Can you work these out from the drawing? Everything is in mm from the part's minimum corner. A direction names the side the tool comes from. Round coordinates to 2 decimals unless told otherwise and drop trailing zeros. Order: outer loops, then holes, each group sorted by start corner. A loop starts at its lowest first (then second) coordinate and runs counter-clockwise, first axis right, second up. Notation, with made-up numbers: M -28,11.5 L 18,11.5 A17 cw 18,25.5 Z; hole C 44,60.25 d2. An arc over 180 degrees is marked long. Write item = value, one per line. Start each with the question number.
Item 1: I want a section at A-A, the plane x = 12. List the corners of the cut face in (y, z) for me.
Item 2: I'm going to push flat-ended pins straight in: P1, Ø3.5, axis at x = 19.79, z = 16.5, coming from the +Y side; P2, Ø1, axis at y = 14, z = 20.5, coming from the -X side; P3, Ø5, axis at x = 4.21, z = 16.5, coming from the -Y side; P4, Ø12, axis at y = 4, z = 18.5, coming from the +X side. Where does each tip first touch, or does it pass through?
Item 3: I want a section at D-D, the plane z = 3. List the corners of the cut face in (x, y) for me, plus the area to 3 significant figures.
Item 4: I want a section at C-C, the plane y = 16.25. List the corners of the cut face in (x, z) for me, plus the area to 3 significant figures.
Item 5: I want a section at B-B, the plane z = 12. List the corners of the cut face in (x, y) for me.
Item 6: For the marked faces 1, 2 and 3, which set-ups out of +Z, -Z, +X, -X, +Y, -Y let a thin tool reach every point of the face, with its end or its side?
Item 7: Please list where these lines run through material, in increasing order: L1, parallel to Z at x = 12, y = 16.05; L2, parallel to X at y = 16.2, z = 16.5 (1 decimal); L3, parallel to Y at x = 2, z = 9.5.
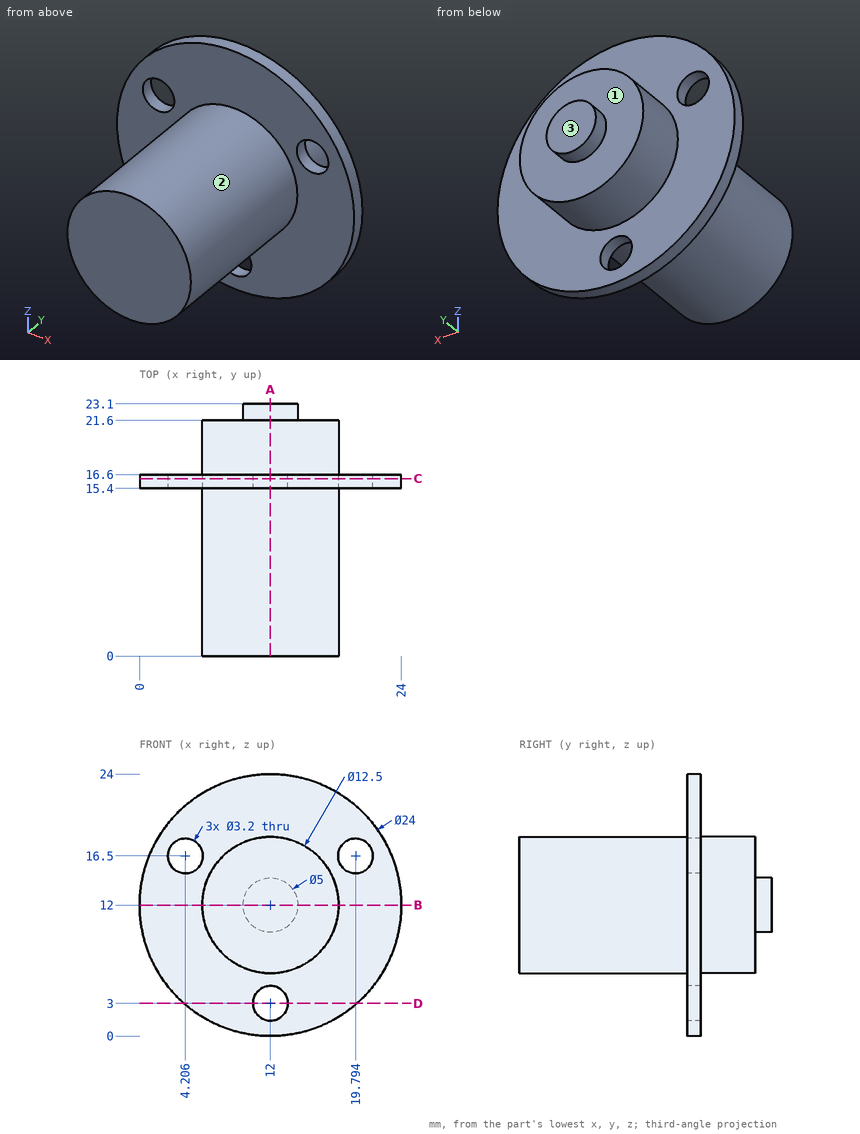
Filled in:
q1.outline = M 0,5.75 L 15.4,5.75 L 15.4,4.6 L 16.6,4.6 L 16.6,5.75 L 21.6,5.75 L 21.6,9.5 L 23.1,9.5 L 23.1,14.5 L 21.6,14.5 L 21.6,18.25 L 16.6,18.25 L 16.6,24 L 15.4,24 L 15.4,18.25 L 0,18.25 Z; M 15.4,0 L 16.6,0 L 16.6,1.4 L 15.4,1.4 Z
q2.P1 = 16.6
q2.P2 = through
q2.P3 = 15.4
q2.P4 = 18.23
q3.outline = M 4.06,15.4 L 10.4,15.4 L 10.4,16.6 L 4.06,16.6 Z; M 13.6,15.4 L 19.94,15.4 L 19.94,16.6 L 13.6,16.6 Z
q3.area = 15.2 mm^2
q4.outline = C 12,12 d24; hole C 4.21,16.5 d3.2; hole C 12,3 d3.2; hole C 19.79,16.5 d3.2
q4.area = 428 mm^2
q5.outline = M 0,15.4 L 5.75,15.4 L 5.75,0 L 18.25,0 L 18.25,15.4 L 24,15.4 L 24,16.6 L 18.25,16.6 L 18.25,21.6 L 14.5,21.6 L 14.5,23.1 L 9.5,23.1 L 9.5,21.6 L 5.75,21.6 L 5.75,16.6 L 0,16.6 Z
q6.face_1 = +Y
q6.face_2 = -Y
q6.face_3 = +Z, -Z, +X, -X, +Y
q7.L1 = 0 to 1.4, 4.6 to 24
q7.L2 = 0.9 to 2.6, 5.8 to 18.2, 21.4 to 23.1
q7.L3 = 15.4 to 16.6
